Design review of the part built by this model. Coordinates are the model's own, in mm. Face numbers are marked on the shaded views. A direction names the side the tool comes from. Round coordinates to 2 decimals unless told otherwise and drop trailing zeros. Write each loop counter-clockwise with the first axis right and the second up, starting at its lowest first coordinate (ties: lowest second). Pieces come first, ordered by that corner, then holes. Notation, with made-up numbers: M -28.75,-29 L -15.75,-29 A12 ccw -15.75,-19 Z; hole C 71,-13 d8. An arc over 180 degrees is marked long. One line per question, with ' | ' between items. Start each with the question number.
Item 1: Add section B-B, the plane x = -12.5. State the section outline as (y, z) points, and give its area (3 significant figures).
Item 2: For L1, parallel to X at y = -2, z = 43; L2, parallel to Y at x = -21, z = 24.5; L3, parallel to Y at x = -22.5, z = 10, list the stretches that pass through material, from the lowest coordinate up.
Item 3: Insertion check: pin 1 Ø1 at (x, z) = (-20, 36.5) entering from +Y; pin 2 Ø0.6 at (x, y) = (-25.5, 16) entering from +Z. Each pin has a flat end and moves straight along its axis. Give the tip position at first contact, or say it passes through.
Item 4: Machinability: for the marked faces 1, 2 and 3, which of the approach directions +Z, -Z, +X, -X, +Y, -Y give a long, thin tool a straight path to every point of the face, cutting with its end or side? Answer none if there is none.
Item 5: Draft analysis for pull direction Y (two halves, no side actions). For the marked faces 4, 5 and 6, state which applies: released by +Y, released by -Y, zero draft, split by the parting line, or undercut.
Item 6: Add section A-A, the plane y = 10. State the section outline as (x, z) points, and give its area (3 significant figures).
Item 7: Add section D-D, the plane x = 28. State the section outline as (y, z) points, and give its area (3 significant figures).
Item 8: Add section C-C, the plane z = 8. State the section outline as (x, y) points.
```python
from build123d import *

# Parameters (mm, degrees)
F1_DEPTH = 75
F2_F1_R  = 1.5
F2_F2_R  = 1.5
F4_W     = 18
F4_H     = 55
F5_DEPTH = 0.5


# Not quite as in the source:
# - a feature names something its author has since deleted; it is built from what else it names


with BuildPart() as f1:
    # F0 (on Top) → F1 (new body)
    with BuildSketch(Plane.XY):
        with BuildLine():
            Line((38, 12.5), (38, -12.5))
            Line((38, -12.5), (-38, -12.5))
            Line((-38, -12.5), (-38, 12.5))
            Line((-38, 12.5), (-7, 12.5))
            ThreePointArc((-7, 12.5), (-5, 14.5), (-7, 16.5))
            Line((-7, 16.5), (-42, 16.5))
            Line((-42, 16.5), (-42, -16.5))
            Line((-42, -16.5), (42, -16.5))
            Line((42, -16.5), (42, 16.5))
            Line((42, 16.5), (7, 16.5))
            ThreePointArc((7, 16.5), (5, 14.5), (7, 12.5))
            Line((7, 12.5), (38, 12.5))
        make_face()
    extrude(amount=F1_DEPTH)

    # F2: fillet of radius 1.5 on 12 edges, made by hand

    # F2_f1
    f2_f1_edges = [f1.edges().sort_by_distance(p)[0] for p in [
        (38, -12.5, 37.5),
        (-38, -12.5, 37.5),
        (-38, 12.5, 37.5),
        (38, 12.5, 37.5),
    ]]
    fillet(f2_f1_edges, radius=F2_F1_R)

    # F2_f2
    f2_f2_edges = [f1.edges().sort_by_distance(p)[0] for p in [
        (0, -12.5, 0),
        (0, -12.5, 75),
        (21.75, 12.5, 0),
        (21.75, 12.5, 75),
        (5, 14.5, 75),
        (24.5, 16.5, 75),
        (5, 14.5, 0),
        (24.5, 16.5, 0),
        (37.5606601718, 12.0606601718, 75),
        (37.5606601718, 12.0606601718, 0),
        (37.5606601718, -12.0606601718, 75),
        (-37.5606601718, -12.0606601718, 75),
        (37.5606601718, -12.0606601718, 0),
        (-37.5606601718, -12.0606601718, 0),
    ]]
    fillet(f2_f2_edges, radius=F2_F2_R)

    # F4 (on offset) → F5 (cut)
    with BuildSketch(Plane(origin=(0, 16.5, 0), x_dir=(-1, 0, 0), z_dir=(0, 1, 0))):
        with Locations((-24.5, 47.5)):
            Rectangle(F4_W, F4_H)
        with Locations((24.5, 47.5)):
            Rectangle(F4_W, F4_H)
    extrude(amount=-F5_DEPTH, mode=Mode.SUBTRACT)


solid = f1.part
```
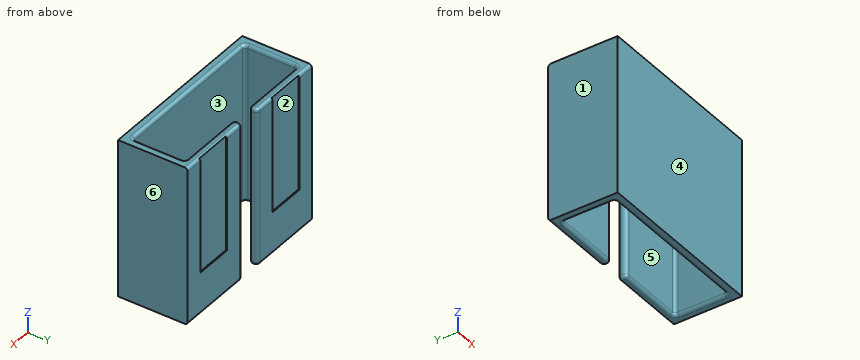
Computed values:
1) outline: M -16.5,0 L -14,0 A1.5 ccw -12.5,1.5 L -12.5,73.5 A1.5 ccw -14,75 L -16.5,75 Z; M 12.5,1.5 A1.5 ccw 14,0 L 15,0 A1.5 ccw 16.5,1.5 L 16.5,73.5 A1.5 ccw 15,75 L 14,75 A1.5 ccw 12.5,73.5 Z | area: 597 mm^2
2) L1: x = -42 to -38, 38 to 42 | L2: y = -16.5 to -12.5, 12.5 to 16 | L3: y = -16.5 to -12.5, 12.5 to 16.5
3) pin 1: stops at y = 16 | pin 2: stops at z = 74.83
4) face 1: +Z, -Z, -X, +Y, -Y | face 2: +Z, +Y | face 3: +Z, -Z
5) face 4: released by -Y | face 5: undercut | face 6: zero draft
6) outline: M -42,0 L -39.5,0 A1.5 ccw -38,1.5 L -38,73.5 A1.5 ccw -39.5,75 L -42,75 Z; M 38,1.5 A1.5 ccw 39.5,0 L 42,0 L 42,75 L 39.5,75 A1.5 ccw 38,73.5 Z | area: 598 mm^2
7) outline: M -16.5,0 L -14,0 A1.5 ccw -12.5,1.5 L -12.5,73.5 A1.5 ccw -14,75 L -16.5,75 Z; M 12.5,1.5 A1.5 ccw 14,0 L 15,0 A1.5 ccw 16.5,1.5 L 16.5,20 L 16,20 L 16,74.62 A1.5 ccw 15,75 L 14,75 A1.5 ccw 12.5,73.5 Z | area: 570 mm^2
8) outline: M -42,-16.5 L 42,-16.5 L 42,16.5 L 7,16.5 A2 ccw 7,12.5 L 36.5,12.5 A1.5 cw 38,11 L 38,-11 A1.5 cw 36.5,-12.5 L -36.5,-12.5 A1.5 cw -38,-11 L -38,11 A1.5 cw -36.5,12.5 L -7,12.5 A2 ccw -7,16.5 L -42,16.5 Z
